Geometry: final body of the model. Coordinates: model frame, mm. Face numbers are marked on the shaded views. Give positions to 0.01 mm unless a question says otherwise; leave off trailing zeros. Write each loop counter-clockwise with the first axis right and the second up, starting at its lowest first coordinate (ties: lowest second). Pieces come first, ordered by that corner, then holes. Notation, with made-up numbers: M -5,63 L 38,63 A21 cw 38,96 Z; hole C 17.5,66.25 d4. An arc over 180 degrees is marked long. Use one line per item in the form item = value. Start each with the question number.
Item 1: Section query B-B on x = 0. Return loops of the section in (y, z).
Item 2: Contact query for flat-ended pins moving along their axis: P1, Ø10, axis at x = -14.29, y = 11.11, coming from the -Z side; P2, Ø5.5, axis at x = 14.29, y = 11.11, coming from the -Z side. Output: stop coordinate, or through.
Item 3: Material intervals for line 1 along Y through (x, z) = (7.75, 3.15); line 2 along Y through (x, z) = (0, 3.1); line 3 along X through (y, z) = (13, 4.35), sorted ascending. Write a range as from..to.
Item 4: Section query A-A on x = 7.75. Return loops of the section in (y, z).
Item 5: Section query C-C on y = 2.5. Return loops of the section in (x, z).
Item 6: Section query D-D on z = 1.6. Give the number of separate pieces and of enclosed holes in the cut face, then the cut area to 3 significant figures.
Item 7: Pull-direction query (Y, two-part tool) for the marked faces 1, 2 and 3; classes: released by +Y, released by -Y, zero draft, split by the parting line, or undercut.
from build123d import *

# Parameters (mm, degrees)
SKETCH1_W                           = 38.1
SKETCH1_H                           = 41.275
BOSS_EXTRUDE1_DEPTH                 = 4.826
SKETCH2_R                           = 7.14375
CUT_EXTRUDE1_DEPTH                  = 29.497353952
F_3_4_3_4_DIAMETER_HOLE1_D          = 3.4
F_1_4_0_25_DIAMETER_HOLE1_D         = 6.35
F_1_8_0_125_CLEARANCE_DOWEL_HOLE1_D = 3.175


with BuildPart() as part:
    # Sketch1 → Boss-Extrude1 (new body)
    with BuildSketch(Plane.XY):
        Rectangle(SKETCH1_W, SKETCH1_H)
    extrude(amount=BOSS_EXTRUDE1_DEPTH)

    # Sketch2 → Cut-Extrude1 (cut, through all)
    with BuildSketch(Plane.XY.offset(4.826)):
        with Locations((0, 10.287)):
            Circle(SKETCH2_R)
    extrude(amount=-CUT_EXTRUDE1_DEPTH, mode=Mode.SUBTRACT)

    # Ø3.4 (3.4) Diameter Hole1 (through all)
    with Locations(Plane.XY.offset(4.826)):
        with Locations((-15.5, 3.287), (7.75, 16.710393759), (15.5, 3.287), (7.75, -10.136393759)):
            Hole(F_3_4_3_4_DIAMETER_HOLE1_D / 2)

    # 1/4 (0.25) Diameter Hole1 (through all)
    with Locations(Plane.XY.offset(4.826)):
        with Locations((-14.2875, 11.1125), (14.2875, 11.1125)):
            Hole(F_1_4_0_25_DIAMETER_HOLE1_D / 2)

    # 1/8 (0.125) Clearance Dowel Hole1 (through all)
    with Locations(Plane.XY.offset(4.826)):
        with Locations((-16.66875, -15.875), (16.66875, -15.875)):
            Hole(F_1_8_0_125_CLEARANCE_DOWEL_HOLE1_D / 2)


solid = part.part
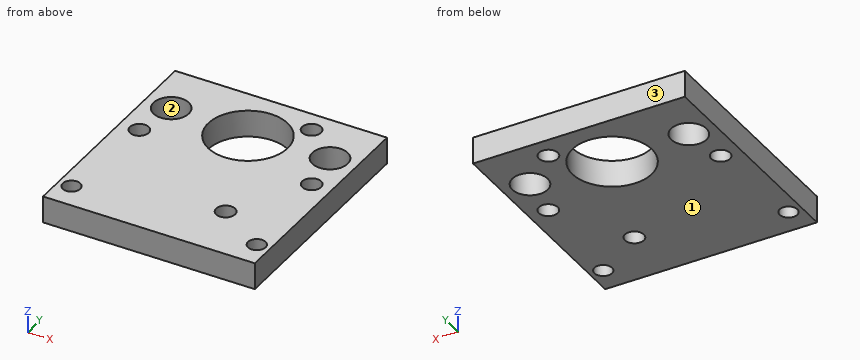
Answer sheet:
q1.outline = M -20.64,0 L 3.14,0 L 3.14,4.83 L -20.64,4.83 Z; M 17.43,0 L 20.64,0 L 20.64,4.83 L 17.43,4.83 Z
q2.P1 = 0
q2.P2 = through
q3.line_1 = -20.64..-11.84, -8.44..15.01, 18.41..20.64
q3.line_2 = -20.64..3.14, 17.43..20.64
q3.line_3 = -19.05..-16.84, -11.73..-6.61, 6.61..11.73, 16.84..19.05
q4.outline = M -20.64,0 L -11.84,0 L -11.84,4.83 L -20.64,4.83 Z; M -8.44,0 L 15.01,0 L 15.01,4.83 L -8.44,4.83 Z; M 18.41,0 L 20.64,0 L 20.64,4.83 L 18.41,4.83 Z
q5.outline = M -19.05,0 L -17.01,0 L -17.01,4.83 L -19.05,4.83 Z; M -13.99,0 L 13.99,0 L 13.99,4.83 L -13.99,4.83 Z; M 17.01,0 L 19.05,0 L 19.05,4.83 L 17.01,4.83 Z
q6.separate_pieces = 1
q6.enclosed_holes = 9
q6.area = 1,300 mm2
q7.face_1 = zero draft
q7.face_2 = undercut
q7.face_3 = released by +Y
